Autodesk Inventor part; units mm, degrees
ref_plane "YZ Plane" through (0, 0, 0) normal (1, 0, 0) x (0, 1, 0)
ref_plane "XZ Plane" through (0, 0, 0) normal (0, 1, 0) x (-1, 0, 0)
ref_plane "XY Plane" through (0, 0, 0) normal (0, 0, 1) x (1, 0, 0)
sketch "Эскиз1" plane through (0, 0, 0) normal (0, 1, 0) x (-1, 0, 0)
  circle A0 centre (0, 0) radius 20
  circle A1 centre (0, 0) radius 10
  circle A2 centre (0, -14) radius 1.5
  circle A3 centre (12.1244, -7) radius 1.5
  circle A4 centre (12.1244, 7) radius 1.5
  circle A5 centre (0, 14) radius 1.5
  circle A6 centre (-12.1244, 7) radius 1.5
  circle A7 centre (-12.1244, -7) radius 1.5
  dimension "d0" = 40
  dimension "d1" = 20
  dimension "d2" = 14
  dimension "d3" = 3
  dimension "d6" = 360
extrude "Выдавливание1" add sketch "Эскиз1" along normal blind 2
properties part number "btnring"
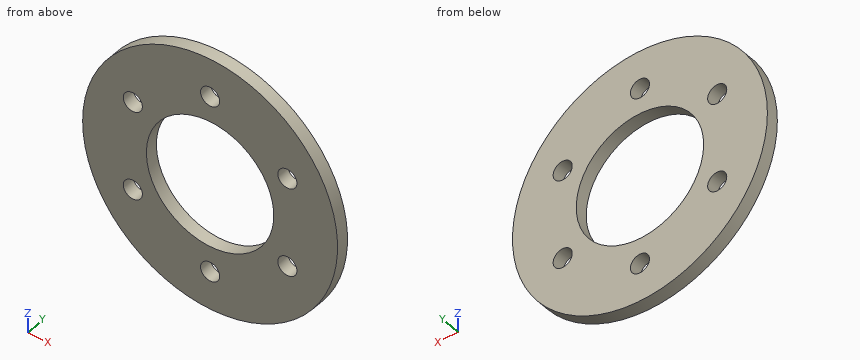
Here's how the part is built. I have some questions about the finished solid (model axes, mm). Round coordinates to 2 decimals unless told otherwise and drop trailing zeros. Order: outer loops, then holes, each group sorted by start corner. A loop starts at its lowest first (then second) coordinate and runs counter-clockwise, first axis right, second up. Notation, with made-up numbers: M 85.25,-13.5 L 118.25,-13.5 A20 ccw 118.25,22.5 Z; hole C -4.75,1.5 d4. An arc over 180 degrees is marked long. Answer as CSV lines item,"result".
Item 1: Imagine slicing it at B-B on x = 0. List the corners of the cut face in (y, z) for me.
From the geometry:
outline,"M 0,-20 L 2,-20 L 2,-15.5 L 0,-15.5 Z; M 0,-12.5 L 2,-12.5 L 2,-10 L 0,-10 Z; M 0,10 L 2,10 L 2,12.5 L 0,12.5 Z; M 0,15.5 L 2,15.5 L 2,20 L 0,20 Z"
Item 2: For pin 1 (4 mm diameter, centred on x = 9.5, z = 13, fed in from -Y); pin 2 (2.5 mm diameter, centred on x = -12.12, z = 7, fed in from +Y) (3 decimals), each with a flat end and sliding along its axis, tell me the tip position at first contact or that it passes through.
From the geometry:
pin 1,"y = 0"
pin 2,"through"
Item 3: Imagine slicing it at C-C on y = 1.25. List the corners of the cut face in (x, z) for me, and give its area (3 significant figures).
From the geometry:
outline,"C 0,0 d40; hole C -12.12,-7 d3; hole C -12.12,7 d3; hole C 0,0 d20; hole C 0,-14 d3; hole C 0,14 d3; hole C 12.12,-7 d3; hole C 12.12,7 d3"
area,"900 mm2"
Item 4: Imagine slicing it at D-D on x = 8.5. List the corners of the cut face in (y, z) for me, and give its area (3 significant figures).
From the geometry:
outline,"M 0,-18.1 L 2,-18.1 L 2,-5.27 L 0,-5.27 Z; M 0,5.27 L 2,5.27 L 2,18.1 L 0,18.1 Z"
area,"51.3 mm2"
Item 5: Please list where these lines run through material, in increasing order: L1, parallel to Z at x = 12.5, y = 0.7; L2, parallel to Z at x = -12, y = 1.3; L3, parallel to X at y = 1.2, z = 13.5. Write a range as [from, to].
From the geometry:
L1,"[-15.61, -8.45], [-5.55, 5.55], [8.45, 15.61]"
L2,"[-16, -8.49], [-5.51, 5.51], [8.49, 16]"
L3,"[-14.76, -1.41], [1.41, 14.76]"
Item 6: Imagine slicing it at A-A on z = 0. List the corners of the cut face in (x, y) for me, and give its area (3 significant figures).
From the geometry:
outline,"M -20,0 L -10,0 L -10,2 L -20,2 Z; M 10,0 L 20,0 L 20,2 L 10,2 Z"
area,"40.0 mm2"
